Input: part model. Units: mm. Frame: model coordinates. A direction names the side the tool comes from. Round coordinates to 2 decimals unless told otherwise and drop trailing zeros. Loops run counter-clockwise (first coordinate to the right, second up) from the corner with the lowest first, then second, coordinate; pieces in that order, holes last. Notation, with made-up numbers: M 27,37.25 L 59,37.25 A15 ccw 59,60.25 Z; hole C 10,10 d8. An arc over 180 degrees is marked long. Return JSON: item names as keys, results as strings. Group by question number.
1) Mould query, pull axis Y, two halves, no side actions, for faces 3 (the face through (-251.744, 425.993, 5.07)), 4 (the face through (246.5, 439.075, 4.93)). Classes: +Y half, -Y half, draft (parallel to the pull), parting line (faces both ways), or undercut.
2) Section A-A (y = 220.5). Output: boundary loops of the cut face in (x, z), plus the area to 3 significant figures.
3) Section C-C (z = 7). Output: boundary loops of the cut face in (x, y), plus the area to 3 significant figures.
4) Access query for faces 1 (the face through (-253.5, 426.95, 4.93)), 2 (the face through (244.792, 438.033, 5.07)). Directions: +Z, -Z, +X, -X, +Y, -Y. A direction counts if a zero-diameter tool reaches every point of the face in a straight line with its end or side. Return the directions, or none.
5) Material intervals for line 1 (X direction, y = 95, z = 8.25); line 2 (Y direction, x = -78.5, z = 1); line 3 (X direction, y = 364, z = 5.75), sorted ascending. Write a range as from..to.
6) Contact query for flat-ended pins moving along their axis: P1, Ø3, axis at x = -31.5, z = 4.5, coming from the +Y side; P2, Ø4, axis at y = 273.5, z = 3.5, coming from the +X side; P3, Ø5, axis at y = 666.5, z = 3.5, coming from the +X side. Output: stop coordinate, or through.
7) Section B-B (x = -120.5). Output: boundary loops of the cut face in (y, z), plus the area to 3 significant figures.
from build123d import *

# Parameters (mm, degrees)
BOSS_EXTRU_1_DEPTH      = 10
ENL_V_MAT_EXTRU_1_DEPTH = 10


with BuildPart() as part:
    # Esquisse1 → Boss.-Extru.1 (new body)
    with BuildSketch(Plane.XY):
        Polygon((-500, 0), (0, 866.025403784), (500, 0), align=None)
    extrude(amount=BOSS_EXTRU_1_DEPTH)

    # Esquisse2 → Enlèv. mat.-Extru.1 (cut)
    with BuildSketch(Plane.XY.offset(10)):
        Polygon((-496.535898385, 2), (0, 862.025403784), (496.535898385, 2), align=None)
    extrude(amount=-ENL_V_MAT_EXTRU_1_DEPTH, mode=Mode.SUBTRACT)


solid = part.part
Returned:
{
 "1": {"face 3": "undercut", "face 4": "+Y half"},
 "2": {"outline": "M -372.69,0 L -370.38,0 L -370.38,10 L -372.69,10 Z; M 370.38,0 L 372.69,0 L 372.69,10 L 370.38,10 Z", "area": "46.2 mm^2"},
 "3": {"outline": "M -500,0 L 500,0 L 0,866.03 Z; hole M -496.54,2 L 496.54,2 L 0,862.03 Z", "area": "5,980 mm^2"},
 "4": {"face 1": "+Z, -Z, -X, +Y", "face 2": "+Z, -Z"},
 "5": {"line 1": "x = -445.15..-442.84, 442.84..445.15", "line 2": "y = 0..2, 726.06..730.06", "line 3": "x = -289.84..-287.54, 287.54..289.84"},
 "6": {"P1": "stops at y = 814.06", "P2": "stops at x = 343.25", "P3": "stops at x = 116.64"},
 "7": {"outline": "M 0,0 L 2,0 L 2,10 L 0,10 Z; M 653.31,0 L 657.31,0 L 657.31,10 L 653.31,10 Z", "area": "60.0 mm^2"}
}
